from build123d import *

# Parameters (mm, degrees)
ESQUISSE3_R                  = 3
ENL_V_MAT_EXTRU_1_DEPTH      = 10
R_P_TITION_CIRCULAIRE1_COUNT = 3


with BuildPart() as part:
    # Esquisse2 → Révolution1 (revolve)
    with BuildSketch(Plane(origin=(0, 0, 0), x_dir=(1, 0, 0), z_dir=(0, 1, 0))):
        with BuildLine():
            Line((-24.196325381, 6), (-24.196325381, 30))
            Line((-24.196325381, 30), (-27.196325381, 30))
            Line((-27.196325381, 30), (-27.196325381, 11))
            ThreePointArc((-27.196325381, 11), (-34.974499974, 7.778174593), (-38.196325381, 0))
            Line((-38.196325381, 0), (-18.196325381, 0))
            ThreePointArc((-18.196325381, 0), (-19.953684694, 4.242640687), (-24.196325381, 6))
        make_face()
    revolve(axis=Axis((-57.66931647, 0, 0), (1, 0, 0)))

    # Esquisse3 → Enlèv. mat.-Extru.1 (cut)
    with BuildSketch(Plane.ZY.offset(27.196325381)):
        with Locations((-22.243253738, -5.851295854)):
            Circle(ESQUISSE3_R)
    enl_v_mat_extru_1 = extrude(amount=-ENL_V_MAT_EXTRU_1_DEPTH, mode=Mode.SUBTRACT)

    # Répétition circulaire1: Enlèv. mat.-Extru.1 ×3 about axis
    r_p_tition_circulaire1_axis = Axis((0, 0, 0), (1, 0, 0))
    for i in range(1, R_P_TITION_CIRCULAIRE1_COUNT):
        add(enl_v_mat_extru_1.rotate(r_p_tition_circulaire1_axis, i * 360 / R_P_TITION_CIRCULAIRE1_COUNT), mode=Mode.SUBTRACT)


solid = part.part
Design review of the part built by this model. Coordinates are the model's own, in mm. A direction names the side the tool comes from. Round coordinates to 2 decimals unless told otherwise and drop trailing zeros. Write each loop counter-clockwise with the first axis right and the second up, starting at its lowest first coordinate (ties: lowest second). Pieces come first, ordered by that corner, then holes. Notation, with made-up numbers: (6.5, 11.5) -> (59.5, 11.5) arc R17 ccw to (59.5, 33.5) -> close; hole circle Ø9 at (15, 78.5). An arc over 180 degrees is marked (long way). One line per question, with ' | ' between items.
(1) Insertion check: P1, Ø8, axis at x = -32.5, y = -19.5, coming from the -Z side; P2, Ø18, axis at y = -7, z = -8, coming from the +X side; P3, Ø4, axis at x = -25, y = 10, coming from the +Z side; P4, Ø3, axis at y = -22, z = -2, coming from the +X side. Each pin has a flat end and moves straight along its axis. Give the tip position at first contact, or say it passes through.
Result sheet:
P1: through | P2: x = -18.42 | P3: z = 28.91 | P4: x = -24.2
(2) Take a section at C-C, the plane z = -21. State the section outline as (x, y) points.
Result sheet:
outline: (-27.2, -21.42) -> (-24.2, -21.42) -> (-24.2, -8.58) -> (-27.2, -8.58) -> close; (-27.2, -3.12) -> (-24.2, -3.12) -> (-24.2, 21.42) -> (-27.2, 21.42) -> close
(3) Take a section at D-D, the plane x = -19.25. State the section outline as (y, z) points, and give its area (3 significant figures).
Result sheet:
outline: circle Ø6.79 at (0, 0) | area: 36.2 mm2
(4) Machinability: for faces 4 (the flat face through (-27.196, -13, 0)), 5 (the cylindrical face through (-25.72, 19.26, 5.4)), which of the approach directions +Z, -Z, +X, -X, +Y, -Y give a long, thin tool a straight path to every point of the face, cutting with its end or side? Answer none if there is none.
Result sheet:
face 4: -X | face 5: +X, -X
(5) Take a section at A-A, the plane z = 0. State the section outline as (x, y) points, and give its area (3 significant figures).
Result sheet:
outline: (-27.2, -30) -> (-24.2, -30) -> (-24.2, -6) arc R6 ccw to (-24.2, 6) -> (-24.2, 30) -> (-27.2, 30) -> (-27.2, 11) arc R11 ccw to (-27.2, -11) -> close | area: 427 mm2
(6) Draft analysis for pull direction Z (two halves, no side actions). For faces 1 (the flat face through (-24.196, 0.4, 6.2)), 2 (the cylindrical face through (-25.72, 1.32, 29.97)), 3 (the cylindrical face through (-25.72, -5.72, -25.24)), state which applies: released by +Z, released by -Z, zero draft, split by the parting line, or undercut.
Result sheet:
face 1: zero draft | face 2: split by the parting line | face 3: undercut
(7) Wall thickness on line 1 (X direction, y = 1, z = 16); line 2 (Z direction, x = -25.75, y = -17); line 3 (Y direction, x = -31.5, z = 4): over which ranges is each line inside the solid? List them lowest first. Write a range as [from, to].
Result sheet:
line 1: [-27.2, -24.2] | line 2: [-24.72, 13.26], [19.11, 24.72] | line 3: [-9.3, 9.3]
